Model file for the job. Use its own axes, mm. A direction names the side the tool comes from. Give positions to 0.01 mm unless a question says otherwise; leave off trailing zeros. Loops run counter-clockwise (first coordinate to the right, second up) from the corner with the lowest first, then second, coordinate; pieces in that order, holes last. Notation, with made-up numbers: (82, 51) -> (98, 51) arc R35 cw to (98, 84) -> close; hole circle Ø6 at (79.5, -25.5). An arc over 180 degrees is marked (long way). Use CSV: the item, a comma, the result in double quotes. Start each with the question number.
(1) Cut at B-B on z = 0. Write the cut outline in (x, y) (3 decimals), then the cut area to 3 significant figures.
(2) Cut at C-C on y = -25. Write the cut outline in (x, z), then the cut area to 3 significant figures.
(3) Cut at A-A on x = 0. Write the cut outline in (y, z) (3 decimals).
(4) 3-axis set-ups, long thin cutter, end or side, ignore diameter. For faces 1 (the flat face through (-1.54, -23.015, 4.42)), 2 (the flat face through (0, -30.015, 0)): which of +Z, -Z, +X, -X, +Y, -Y reach the whole face in a straight line?
(5) Flat gauge pins, fed straight in: pin 1 (5 mm diameter, centred on y = -21.5, z = -3, fed in from -X); pin 2 (1.5 mm diameter, centred on y = -26.5, z = 6, fed in from -X); pin 3 (4 mm diameter, centred on x = 0, y = -21.5, fed in from +Z). Where does each tip first touch, or does it go through?
(6) Cut at D-D on y = -21.75. Write the cut outline in (x, z), then the cut area to 3 significant figures.
(7) Drill centre lines: probe 1 along Y at (x, z) = (-5, -2) (3 decimals); probe 2 along Z at (x, y) = (0.25, -26.25); probe 3 along X at (y, z) = (-25.5, 3). Where is each one in solid material? Low to high.
from build123d import *

# Parameters (mm, degrees)
FILLET2_R = 1.5


with BuildPart() as part:
    # Sketch2 → Revolve1 (revolve)
    with BuildSketch(Plane.XY):
        Polygon((0, -30.015007431), (8, -30.015007431), (8, -23.015007431), (4.5, -23.015007431), (4.5, -22.015007431), (1.5, -20.015007431), (1.5, -18.015007431), (0, -18.015007431), align=None)
    revolve(axis=Axis((0, 46.076216781, 0), (0, -1, 0)))

    # Fillet2
    fillet2_edges = [part.edges().sort_by_distance(p)[0] for p in [
        (-8, -23.015007431, 0),
    ]]
    fillet(fillet2_edges, radius=FILLET2_R)


solid = part.part
Check result:
1,outline,"(-8, -30.015) -> (8, -30.015) -> (8, -24.515) arc R1.5 ccw to (6.5, -23.015) -> (4.5, -23.015) -> (4.5, -22.015) -> (1.5, -20.015) -> (1.5, -18.015) -> (-1.5, -18.015) -> (-1.5, -20.015) -> (-4.5, -22.015) -> (-4.5, -23.015) -> (-6.5, -23.015) arc R1.5 ccw to (-8, -24.515) -> close"
1,area,"138 mm²"
2,outline,"circle Ø16 at (0, 0)"
2,area,"201 mm²"
3,outline,"(-30.015, -8) -> (-24.515, -8) arc R1.5 ccw to (-23.015, -6.5) -> (-23.015, -4.5) -> (-22.015, -4.5) -> (-20.015, -1.5) -> (-18.015, -1.5) -> (-18.015, 1.5) -> (-20.015, 1.5) -> (-22.015, 4.5) -> (-23.015, 4.5) -> (-23.015, 6.5) arc R1.5 ccw to (-24.515, 8) -> (-30.015, 8) -> close"
4,face 1,"+Y"
4,face 2,"+Z, -Z, +X, -X, -Y"
5,pin 1,"x = -7.55"
5,pin 2,"x = -6.04"
5,pin 3,"z = 7.6"
6,outline,"circle Ø8.2 at (0, 0)"
6,area,"52.9 mm²"
7,probe 1,"-30.015 to -23.015"
7,probe 2,"-8 to 8"
7,probe 3,"-7.42 to 7.42"
